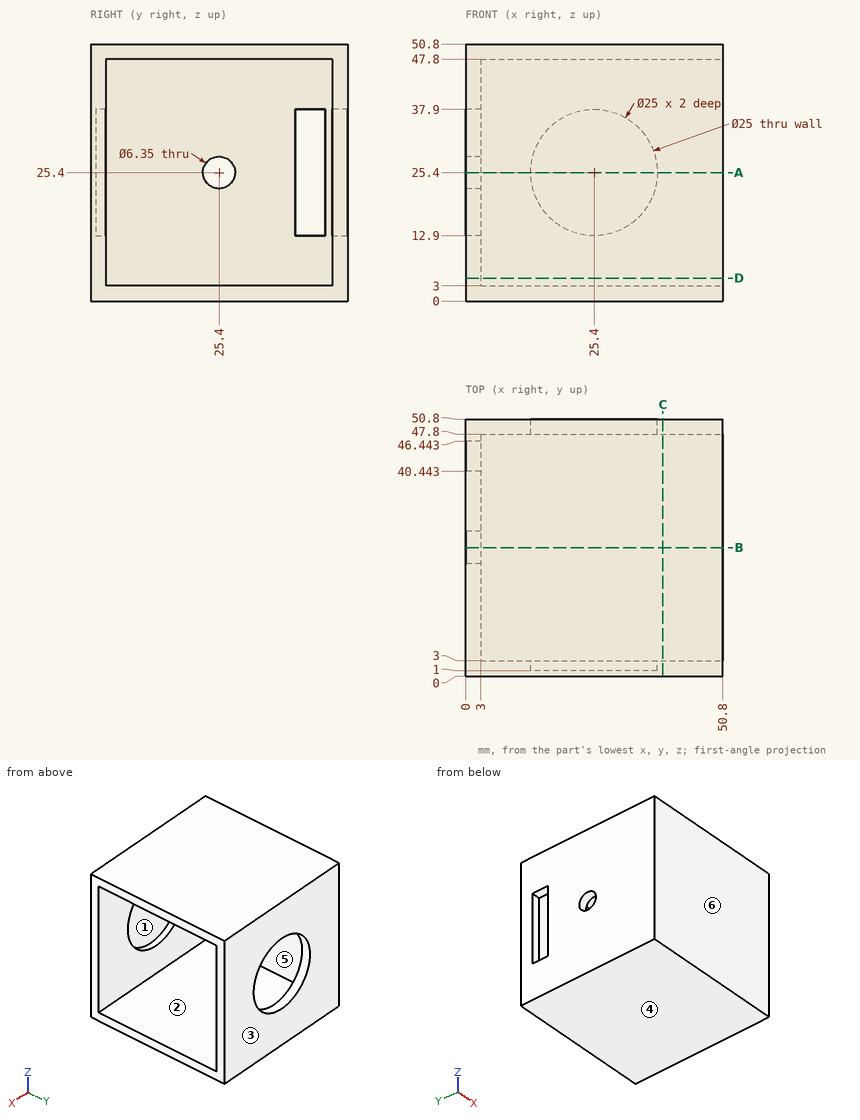
Design review of the part shown in the three views and the two pictorial views. Dimensions are in mm from the part's minimum x, y and z. A direction names the side the tool comes from. Give positions to 0.01 mm unless a question says otherwise; leave off trailing zeros. Write each loop counter-clockwise with the first axis right and the second up, starting at its lowest first coordinate (ties: lowest second). Pieces come first, ordered by that corner, then holes.
(1) Add section D-D (z = 4.5). Give the boundary of the cut face in (x, y).
Checked values:
outline: (0, 0) - (50.8, 0) - (50.8, 3) - (3, 3) - (3, 47.8) - (50.8, 47.8) - (50.8, 50.8) - (0, 50.8) - close
(2) Tool access review of the marked faces 1, 2 and 3: name each direction out of +Z, -Z, +X, -X, +Y, -Y from which nothing blocks a thin tool from reaching the whole face with its end or side.
Checked values:
face 1: +Y
face 2: +X
face 3: +Z, -Z, +X, -X, +Y
(3) Clearance check with flat-ended pins moving along their axes: pin 1 Ø5 at (y, z) = (25.4, 25.4) entering from -X; pin 2 Ø12 at (y, z) = (38, 17.5) entering from +X; pin 3 Ø7.5 at (x, z) = (20.5, 28) entering from +Y. State where each tip first meets the part, or that it passes through.
Checked values:
pin 1: passes through
pin 2: stops at x = 3
pin 3: stops at y = 1
(4) Add section A-A (z = 25.4). Give the boundary of the cut face in (x, y) (1 decimal), and give its area (3 significant figures).
Checked values:
outline: (0, 0) - (50.8, 0) - (50.8, 3) - (37.9, 3) - (37.9, 1) - (12.9, 1) - (12.9, 3) - (3, 3) - (3, 22.2) - (0, 22.2) - close; (0, 28.6) - (3, 28.6) - (3, 40.4) - (0, 40.4) - close; (0, 46.4) - (3, 46.4) - (3, 47.8) - (12.9, 47.8) - (12.9, 50.8) - (0, 50.8) - close; (37.9, 47.8) - (50.8, 47.8) - (50.8, 50.8) - (37.9, 50.8) - close
area: 277 mm2
(5) Add section B-B (y = 25.4). Give the boundary of the cut face in (x, z) (1 decimal).
Checked values:
outline: (0, 0) - (50.8, 0) - (50.8, 3) - (3, 3) - (3, 22.2) - (0, 22.2) - close; (0, 28.6) - (3, 28.6) - (3, 47.8) - (50.8, 47.8) - (50.8, 50.8) - (0, 50.8) - close
(6) Wall thickness on line 1 along X through (y, z) = (49, 25); line 2 along Y through (x, z) = (47, 21): over which ranges is each line inside the solid? List them lowest first.
Checked values:
line 1: x = 0 to 12.91, 37.89 to 50.8
line 2: y = 0 to 3, 47.8 to 50.8
(7) Mouldability with a two-part tool opening along Z and no side actions: class the marked faces 4, 5 and 6 as +Z half, -Z half, draft (parallel to the pull), parting line (faces both ways), or undercut.
Checked values:
face 4: -Z half
face 5: undercut
face 6: draft
(8) Add section C-C (x = 39). Give the boundary of the cut face in (y, z).
Checked values:
outline: (0, 0) - (50.8, 0) - (50.8, 50.8) - (0, 50.8) - close; hole (3, 3) - (47.8, 3) - (47.8, 47.8) - (3, 47.8) - close
